```python
from build123d import *

# Parameters (mm, degrees)
SKETCH_W         = 120
SKETCH_H         = 200
PAD_DEPTH        = 7
HOLE_D           = 5.5
HOLE_CSINK_D     = 11
HOLE_CSINK_ANGLE = 90
SKETCH002_R      = 2.25
HOLE001_DEPTH    = 7.001
SKETCH003_W      = 10
SKETCH003_H      = 5
PAD001_DEPTH     = 8
SKETCH004_R      = 11.2
SKETCH004_R_2    = 1.7
POCKET_DEPTH     = 13
SKETCH005_W      = 4
SKETCH005_H      = 50
PAD002_DEPTH     = 20
PAD009_DEPTH     = 3
PAD010_DEPTH     = 3
SKETCH019_W      = 11
SKETCH019_H      = 9
SKETCH019_W_2    = 7.2
SKETCH019_H_2    = 3.2
PAD011_DEPTH     = 8
SKETCH020_R      = 2
POCKET001_DEPTH  = 14
SKETCH022_W      = 18
SKETCH022_H      = 31
PAD012_DEPTH     = 5
PAD013_DEPTH     = 4
SKETCH024_R      = 2.5
POCKET003_DEPTH  = 7
SKETCH026_W      = 23
SKETCH026_H      = 20
PAD014_DEPTH     = 20
SKETCH030_R      = 2.1
POCKET004_DEPTH  = 7
SKETCH031_R      = 1.6
POCKET005_DEPTH  = 5
SKETCH032_W      = 14
SKETCH032_H      = 16
POCKET006_DEPTH  = 20
SKETCH034_R      = 2.1
POCKET008_DEPTH  = 120
SKETCH035_R      = 2.239489
POCKET009_DEPTH  = 12
FILLET_R         = 3
FILLET001_R      = 4
FILLET002_R      = 6
FILLET003_R      = 4


with BuildPart() as part:
    # Sketch → Pad (new body)
    with BuildSketch(Plane.XY):
        with Locations((-10, 100)):
            Rectangle(SKETCH_W, SKETCH_H)
    extrude(amount=PAD_DEPTH)

    # Hole (through all)
    with Locations(Plane.XY.offset(7)):
        with Locations((17, 7), (17, 43), (-17, 43), (-17, 7), (12, 115), (12, 75), (-12, 115), (-12, 75)):
            CounterSinkHole(HOLE_D / 2, HOLE_CSINK_D / 2, counter_sink_angle=HOLE_CSINK_ANGLE)

    # Sketch002 (on Face5 of Hole) → Hole001 (cut, through all)
    with BuildSketch(Plane.XY.offset(7)):
        with Locations((0, 10)):
            Circle(SKETCH002_R)
        with Locations((0, 50)):
            Circle(SKETCH002_R)
        with Locations((0, 90)):
            Circle(SKETCH002_R)
        with Locations((0, 130)):
            Circle(SKETCH002_R)
        with Locations((0, 170)):
            Circle(SKETCH002_R)
    extrude(amount=-HOLE001_DEPTH, mode=Mode.SUBTRACT)

    # Sketch003 (on Face5 of Hole001) → Pad001 (join)
    with BuildSketch(Plane.XY.offset(7)):
        with Locations((-2e-06, 2.5)):
            Rectangle(SKETCH003_W, SKETCH003_H)
    extrude(amount=PAD001_DEPTH)

    # Sketch004 (on Face5 of Pad001) → Pocket (cut)
    with BuildSketch(Plane.XY.offset(7)):
        with Locations((-48, 177)):
            Circle(SKETCH004_R)
        with Locations((-63.5, 192.5)):
            Circle(SKETCH004_R_2)
        with Locations((-32.5, 192.5)):
            Circle(SKETCH004_R_2)
        with Locations((-32.5, 161.5)):
            Circle(SKETCH004_R_2)
        with Locations((-63.5, 161.5)):
            Circle(SKETCH004_R_2)
        with BuildLine():
            ThreePointArc((-50.6, 10), (-48, 7.4), (-45.4, 10))
            Line((-45.4, 10), (-45.4, 20))
            ThreePointArc((-45.4, 20), (-48, 22.6), (-50.6, 20))
            Line((-50.6, 20), (-50.6, 10))
        make_face()
    extrude(amount=-POCKET_DEPTH, mode=Mode.SUBTRACT)

    # Sketch005 (on DatumPlane) → Pad002 (join)
    with BuildSketch(Plane.XY.offset(7)):
        with Locations((-68, 82)):
            Rectangle(SKETCH005_W, SKETCH005_H)
        with Locations((48, 82)):
            Rectangle(SKETCH005_W, SKETCH005_H)
    extrude(amount=PAD002_DEPTH)

    # Sketch017 (on DatumPlane) → Pad009 (join)
    with BuildSketch(Plane(origin=(0, 107, 0), x_dir=(-1, 0, 0), z_dir=(0, 1, 0))):
        Polygon((66, 7), (66, 27), (56, 7), align=None)
        Polygon((-46, 27), (-46, 7), (-36, 7), align=None)
    extrude(amount=-PAD009_DEPTH)

    # Sketch018 (on DatumPlane) → Pad010 (join)
    with BuildSketch(Plane.XZ.offset(-57)):
        Polygon((-66, 7), (-66, 27), (-56, 7), align=None)
        Polygon((46, 7), (46, 26.679939), (36, 7), align=None)
    extrude(amount=-PAD010_DEPTH)

    # Sketch019 (on Face5 of Pad010) → Pad011 (join)
    with BuildSketch(Plane.XY.offset(7)):
        with Locations((-48, 42.132326)):
            Rectangle(SKETCH019_W, SKETCH019_H)
        with Locations((-48, 42.232326)):
            Rectangle(SKETCH019_W_2, SKETCH019_H_2, mode=Mode.SUBTRACT)
    extrude(amount=PAD011_DEPTH)

    # Sketch020 → Pocket001 (cut)
    with BuildSketch(Plane(origin=(0, 50.499198, 0), x_dir=(-1, 0, 0), z_dir=(0, 1, 0))):
        with Locations((28, 12)):
            Circle(SKETCH020_R)
    extrude(amount=-POCKET001_DEPTH, mode=Mode.SUBTRACT)

    # Sketch022 (on DatumPlane) → Pad012 (join)
    with BuildSketch(Plane(origin=(0, 200, 0), x_dir=(-1, 0, 0), z_dir=(0, 1, 0))):
        with Locations((0, 15.5)):
            Rectangle(SKETCH022_W, SKETCH022_H)
    extrude(amount=-PAD012_DEPTH)

    # Sketch023 (on DatumPlane) → Pad013 (join)
    with BuildSketch(Plane.YZ.offset(9)):
        Polygon((200, 7), (189, 7), (195, 31), (200, 31), align=None)
    extrude(amount=PAD013_DEPTH)

    # Sketch024 (on Face5 of Pad013) → Pocket003 (cut)
    with BuildSketch(Plane.XY.offset(7)):
        with Locations((0, 189.428879)):
            Circle(SKETCH024_R)
    extrude(amount=-POCKET003_DEPTH, mode=Mode.SUBTRACT)

    # Sketch026 (on DatumPlane) → Pad014 (join)
    with BuildSketch(Plane.YZ.offset(50)):
        with Locations((188.5, 10)):
            Rectangle(SKETCH026_W, SKETCH026_H)
    extrude(amount=PAD014_DEPTH)

    # Sketch030 → Pocket004 (cut)
    with BuildSketch(Plane.XY.offset(7)):
        with Locations((21.000004, 193.991192)):
            Circle(SKETCH030_R)
        with Locations((29.000004, 193.989173)):
            Circle(SKETCH030_R)
        with Locations((37.000002, 193.994382)):
            Circle(SKETCH030_R)
        with Locations((45, 194)):
            Circle(SKETCH030_R)
    extrude(amount=-POCKET004_DEPTH, mode=Mode.SUBTRACT)

    # Sketch031 (on Face90 of Pocket004) → Pocket005 (cut)
    with BuildSketch(Plane(origin=(0, 200, 0), x_dir=(-1, 0, 0), z_dir=(0, 1, 0))):
        with Locations((-6, 11)):
            Circle(SKETCH031_R)
        with Locations((6, 11)):
            Circle(SKETCH031_R)
    extrude(amount=-POCKET005_DEPTH, mode=Mode.SUBTRACT)

    # Sketch032 (on Face86 of Pocket005) → Pocket006 (cut)
    with BuildSketch(Plane(origin=(0, 200, 0), x_dir=(-1, 0, 0), z_dir=(0, 1, 0))):
        with Locations((-60, 10)):
            Rectangle(SKETCH032_W, SKETCH032_H)
    extrude(amount=-POCKET006_DEPTH, mode=Mode.SUBTRACT)

    # Sketch034 (on DatumPlane) → Pocket008 (cut)
    with BuildSketch(Plane(origin=(-70, 0, 0), x_dir=(0, -1, 0), z_dir=(-1, 0, 0))):
        with Locations((-99, 17)):
            Circle(SKETCH034_R)
        with Locations((-82, 17)):
            Circle(SKETCH034_R)
        with Locations((-65, 17)):
            Circle(SKETCH034_R)
    extrude(amount=-POCKET008_DEPTH, mode=Mode.SUBTRACT)

    # Sketch035 (on Face55 of Pad011) → Pocket009 (cut)
    with BuildSketch(Plane(origin=(0, 46.632326, 0), x_dir=(-1, 0, 0), z_dir=(0, 1, 0))):
        with Locations((47.996092, 10.986399)):
            Circle(SKETCH035_R)
    extrude(amount=-POCKET009_DEPTH, mode=Mode.SUBTRACT)

    # Fillet
    fillet_edges = [part.edges().sort_by_distance(p)[0] for p in [
        (-9, 197.5, 31),
        (13, 197.5, 31),
    ]]
    fillet(fillet_edges, radius=FILLET_R)

    # Fillet001
    fillet001_edges = [part.edges().sort_by_distance(p)[0] for p in [
        (50, 188.5, 20),
        (70, 188.5, 20),
        (70, 188.5, 0),
    ]]
    fillet(fillet001_edges, radius=FILLET001_R)

    # Fillet002
    fillet002_edges = [part.edges().sort_by_distance(p)[0] for p in [
        (-70, 200, 3.5),
        (50, 0, 3.5),
        (-70, 0, 3.5),
    ]]
    fillet(fillet002_edges, radius=FILLET002_R)

    # Fillet003
    fillet003_edges = [part.edges().sort_by_distance(p)[0] for p in [
        (-5.000002, 2.5, 15),
        (4.999998, 2.5, 15),
    ]]
    fillet(fillet003_edges, radius=FILLET003_R)


solid = part.part
```
The listing builds one solid part. Answer for the finished solid, in the listing's coordinates (mm). A direction names the side the tool comes from. Coordinates: 2 decimals unless noted, no trailing zeros. Loops run counter-clockwise (first coordinate to the right, second up) from the corner with the lowest first, then second, coordinate; pieces in that order, holes last. Notation, with made-up numbers: (78.5, 3.25) -> (113.5, 3.25) arc R27 cw to (113.5, 29.25) -> close; hole circle Ø3 at (49, -14.5). An arc over 180 degrees is marked (long way). Return JSON: item names as keys, results as strings. Group by question number.
(1) Find the intervals of material crossed by probe 1 along X at (y, z) = (7, 2); probe 2 along X at (y, z) = (68.5, 16.5); probe 3 along Y at (x, z) = (-60, 7.5), in increasing order. Write a range as from..to.
(2) Which of the six approach directions +Z, -Z, +X, -X, +Y, -Y give full straight-line access (tool end or side, diameter ignored) to faces 4 (the flat face through (-42.5, 42, 11)), 5 (the flat face through (-61, 58, 17)), 6 (the cylindrical face through (-0.29, 52.23, 3.55)), 7 (the flat face through (0, 5, 11)), 8 (the cylindrical face through (-50.065, 45.252, 10.129))?
(3) A cutting plane is placed at B-B on z = 22.5. Write down the section's boundary in (x, y) (3 decimals), and give its area (3 significant figures).
(4) A cutting plane is placed at A-A on y = 99. Write down the section's boundary in (x, z).
(5) Determine the mould class of faces 1 (the cylindrical face through (-50.065, 39.153, 10.129)), 2 (the cylindrical face through (-0.488, 167.804, 3.549)), 3 (the flat face through (44, 107, 15)) for opening direction Y: released by +Y, released by -Y, zero draft, split by the parting line, or undercut.
(6) Given pin 1 Ø1.5 at (y, z) = (177.5, 17) entering from +X; pin 2 Ø5 at (y, z) = (82, 17) entering from +X; pin 3 Ø2 at (x, z) = (43.5, 10.5) entering from +Y; pin 4 Ø12 at (y, z) = (48, 21) entering from -X, each flat-ended and moving along its own axis, determine where each tip first touches the part or whether it passes through.
The answers:
{
 "1": {"probe 1": "x = -70..-19.75, -14.25..14.25, 19.75..50", "probe 2": "x = -70..-66, 46..50", "probe 3": "y = 57..60, 104..107"},
 "2": {"face 4": "+Z, +X, +Y, -Y", "face 5": "+Z, +Y, -Y", "face 6": "+Z, -Z", "face 7": "+Z, +X, -X", "face 8": "+Y, -Y"},
 "3": {"outline": "(-70, 57) -> (-63.75, 57) -> (-63.75, 60) -> (-66, 60) -> (-66, 104) -> (-63.75, 104) -> (-63.75, 107) -> (-70, 107) -> close; (-9, 195) -> (9, 195) -> (9, 192.875) -> (13, 192.875) -> (13, 200) -> (-9, 200) -> close; (43.75, 104) -> (46, 104) -> (46, 60) -> (43.876, 60) -> (43.876, 57) -> (50, 57) -> (50, 107) -> (43.75, 107) -> close", "area": "545 mm^2"},
 "4": {"outline": "(-70, 0) -> (50, 0) -> (50, 14.9) -> (46, 14.9) -> (46, 7) -> (-66, 7) -> (-66, 14.9) -> (-70, 14.9) -> close; (-70, 19.1) -> (-66, 19.1) -> (-66, 27) -> (-70, 27) -> close; (46, 19.1) -> (50, 19.1) -> (50, 27) -> (46, 27) -> close"},
 "5": {"face 1": "zero draft", "face 2": "undercut", "face 3": "released by +Y"},
 "6": {"pin 1": "stops at x = 69.99", "pin 2": "stops at x = 50", "pin 3": "stops at y = 107", "pin 4": "passes through"}
}
